from build123d import *

# Parameters (mm, degrees)
FILLET1_R          = 0.381
CHAMFER1_SIZE      = 0.381
FILLET2_R          = 0.8128
CUT_EXTRUDE1_DEPTH = 2.54


with BuildPart() as part:
    # Sketch1 → Revolve1 (revolve)
    with BuildSketch(Plane.XY, mode=Mode.PRIVATE) as revolve1_sk:
        with BuildLine():
            Line((0, -15.875), (-1.905, -15.875))
            Line((-1.905, -15.875), (-1.905, -3.661588624))
            ThreePointArc((-1.905, -3.661588624), (-4.009330573, 0.980573609), (0, 4.1275))
            Line((0, 4.1275), (0, -15.875))
        make_face()
    revolve(revolve1_sk.sketch.rotate(Axis((0, -648.634401367, 0), (0, 1, 0)), 180), axis=Axis((0, -648.634401367, 0), (0, 1, 0)))

    # Fillet1
    fillet1_edges = [part.edges().sort_by_distance(p)[0] for p in [
        (-1.905, -3.661588624, 0),
    ]]
    fillet(fillet1_edges, radius=FILLET1_R)

    # Chamfer1
    chamfer1_edges = [part.edges().sort_by_distance(p)[0] for p in [
        (-1.905, -15.875, 0),
    ]]
    chamfer(chamfer1_edges, length=CHAMFER1_SIZE)

    # Split1
    split(bisect_by=Plane.ZX.offset(3.574519854), keep=Keep.BOTTOM)

    # Fillet2
    fillet2_edges = [part.edges().sort_by_distance(p)[0] for p in [
        (-2.06375, 3.574519854, 0),
    ]]
    fillet(fillet2_edges, radius=FILLET2_R)

    # Sketch3 → Cut-Extrude1 (cut)
    with BuildSketch(Plane(origin=(0, 3.574519854, 0), x_dir=(1, 0, 0), z_dir=(0, 1, 0))):
        Polygon((0.687407664, 1.190625), (-0.687407664, 1.190625), (-1.374815329, 0), (-0.687407664, -1.190625), (0.687407664, -1.190625), (1.374815329, 0), align=None)
    extrude(amount=-CUT_EXTRUDE1_DEPTH, mode=Mode.SUBTRACT)


solid = part.part
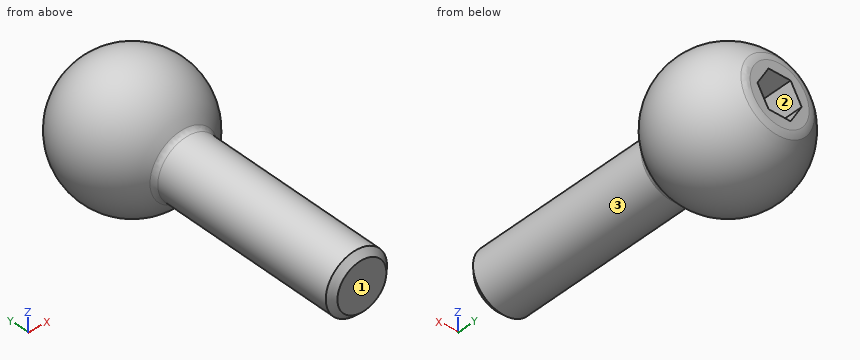
CAD build for the part. Positions are in the model's coordinates, mm. Face numbers are marked on the shaded views. Give positions to 0.01 mm unless a question says otherwise; leave off trailing zeros. Loops run counter-clockwise (first coordinate to the right, second up) from the corner with the lowest first, then second, coordinate; pieces in that order, holes last. Notation, with made-up numbers: M -10,-8.75 L 41,-8.75 A3 cw 41,-4.75 Z; hole C 79.25,14.25 d2. An arc over 180 degrees is marked long. One line per question, with ' | ' between items. Start each with the question number.
1. Probe L1, parallel to X at y = -13.25, z = 0.5; L2, parallel to Y at x = 0.25, z = 0.75 (3 decimals); L3, parallel to Y at x = -2.5, z = 3. List the from-to ranges inside material, lowest first. Write a range as from..to.
2. Saw through at B-B on y = -11.5. Give the cut face in (x, z) (3 decimals).
3. Saw through at C-C on x = -2.75. Give the cut face in (y, z), plus the area to 3 significant figures.
4. Two-plate mould, pull along Z, no slides. Class the marked faces 1, 2 and 3: pulls with the +Z half, pulls with the -Z half, needs draft (parallel to the pull), parting line crosses it, or undercut.
5. Flat gauge pins, fed straight in: pin 1 (1.5 mm diameter, centred on x = 1.5, y = -7, fed in from -Z); pin 2 (1.1 mm diameter, centred on x = 0, y = 2, fed in from -Z); pin 3 (0.7 mm diameter, centred on x = 0, y = 2, fed in from +Z); pin 4 (1 mm diameter, centred on x = -3, y = -8.5, fed in from +Z). Where does each tip first touch, or does it go through?
6. Saw through at A-A on y = 2.25. Give the cut face in (x, z).
Result sheet:
1) L1: x = -1.84..1.84 | L2: y = -15.875..1.035 | L3: y = -1.34..1.34
2) outline: C 0,0 d3.81
3) outline: C 0,0 d6.16 | area: 29.8 mm^2
4) face 1: needs draft | face 2: undercut | face 3: parting line crosses it
5) pin 1: stops at z = -1.75 | pin 2: stops at z = -3.86 | pin 3: stops at z = 3.78 | pin 4: passes through
6) outline: C 0,0 d6.92; hole M -1.37,0 L -0.69,-1.19 L 0.69,-1.19 L 1.37,0 L 0.69,1.19 L -0.69,1.19 Z
